Solid Edge part; units mm, degrees
sketch "Sketch1" plane through (0, 0, 0) normal (0, 0, 1) x (1, 0, 0)
  circle A0 centre (0, 0) radius 4.25
extrude "Protrusion1" add sketch "Sketch1" along normal blind 5
sketch "Sketch2" plane through (0, 0, 5) normal (0, 0, 1) x (0, 1, 0)
  line L0 (0, 2.3094) -> (2, 1.1547)
  line L1 (2, 1.1547) -> (2, -1.1547)
  line L2 (2, -1.1547) -> (0, -2.3094)
  line L3 (0, -2.3094) -> (-2, -1.1547)
  line L4 (-2, -1.1547) -> (-2, 1.1547)
  line L5 (-2, 1.1547) -> (0, 2.3094)
extrude "Cutout1" cut sketch "Sketch2" against normal blind 2.5
fillet "Round1" radius 0.5 1 edges at (-4.25, 0, 5)
sketch "Sketch3" plane through (0, 0, 0) normal (1, 0, 0) x (0, 1, 0)
  line L0 (-2.0095, -10) -> (0, -10)
  line L1 (-2.5, -9.5095) -> (-2.0095, -10)
  line L2 (-2.5, -2.4) -> (-2.5, -9.5095)
  line L3 (-2.0095, -2.4) -> (-2.5, -2.4)
  line L4 (-2.0095, -2.39) -> (-2.0095, -2.4)
  line L5 (-2.5, -2.39) -> (-2.0095, -2.39)
  line L6 (-2.5, -0.2) -> (-2.5, -2.39)
  arc A0 (-2.5, -0.2) -> (-2.7, 0) centre (-2.7, -0.2) ccw
revolve "RevolvedProtrusion1" add sketch "Sketch3" angle 360 about axis through (0, 0, -60.325) along (0, 0, 1) material side at (0, -1.0048, -9.95)
cosmetic_thread "Thread1"
sketch "Sketch4" plane through (0, 0, 0) normal (0, -1, 0) x (1, 0, 0)
  line L0 (-2.29, 5) -> (0, 3.6779)
revolve "RevolvedCutout1" cut sketch "Sketch4" angle 360 about axis through (0, 0, 57.15) along (0, 0, -1) material side at (-1.12, 0, 4.3823)
properties material "Stahl"
Verification items for the finished model (mm, model axes). A direction names the side the tool comes from. Coordinates: 2 decimals unless noted, no trailing zeros. Order: outer loops, then holes, each group sorted by start corner. A loop starts at its lowest first (then second) coordinate and runs counter-clockwise, first axis right, second up.
1. Go/stop test with flat-tipped pins: pin 1 Ø3 at (x, y) = (-1, -0.5) entering from +Z; pin 2 Ø1 at (y, z) = (2, -4) entering from -X; pin 3 Ø3 at (x, z) = (-1, -5.5) entering from -Y; pin 4 Ø1 at (y, z) = (0, -5.5) entering from +X. Record where each tip stops, or that it passes through.
Results found:
pin 1: stops at z = 5
pin 2: stops at x = -2
pin 3: stops at y = -2.5
pin 4: stops at x = 2.5
2. Sectioned sample at B-B, the plane z = -1. Record the cut outline in (x, y), and give its area (3 significant figures).
Results found:
outline: circle Ø5 at (0, 0)
area: 19.6 mm2
3. Set-up check for faces 1 (the face through (2.285, -3.584, 2.218)), 2 (the face through (1.724, 1.014, 3.768)), 3 (the face through (2.44, 0.54, -1.31)): record each of +Z, -Z, +X, -X, +Y, -Y from which the full face is reachable in a straight line by a thin tool's end or side.
Results found:
face 1: +Z, -Z
face 2: +Z
face 3: -Z
4. Scan lines: line 1 (X direction, y = 1, z = -4); line 2 (Z direction, x = 0, y = 0.5); line 3 (Z direction, x = -3, y = 1). Record each from-to range of solid material in increasing order.
Results found:
line 1: x = -2.29 to 2.29
line 2: z = -10 to 2.5
line 3: z = 0 to 5
